The model under review builds one solid part; all positions refer to its coordinate system, in mm. A direction names the side the tool comes from. Round coordinates to 2 decimals unless told otherwise and drop trailing zeros. Order: outer loops, then holes, each group sorted by start corner. A loop starts at its lowest first (then second) coordinate and runs counter-clockwise, first axis right, second up. Notation, with made-up numbers: M 29.5,29.5 L 39.5,29.5 A17 ccw 39.5,45.5 Z; hole C 66,50.25 d1. An arc over 180 degrees is marked long. Use a Markdown table: item, result. Add a question column.
1. The part is to be moulded in two halves that separate along X. For faces 1 (the cylindrical face through (105.86, 32.29, 1.62)), 2 (the flat face through (72, 50, 3.2)), 3 (the cylindrical face through (2.795, 79.649, 1.623)), 4 (the flat face through (145.885, 49, 2)), say which applies: +X half, -X half, draft (parallel to the pull), parting line (faces both ways), or undercut.
2. Consider section B-B on x = 53. State the section outline as (y, z) points (3 decimals).
3. Insertion check: P1, Ø1.4, axis at x = 85.34, y = 46.7, coming from the +Z side (3 decimals). The pin has a flat end and moves straight along its axis. Give the tip position at first contact, or say it passes through.
4. To check wall thickness, follow probe 1 along X at (y, z) = (14, 1.6); probe 2 along X at (y, z) = (56.5, 0.85); probe 3 along Y at (x, z) = (26, 2.65) (3 decimals). State the ranges of each line that lie inside material, in increasing order.
5. For faces 5 (the flat face through (0, 49, 2)), 6 (the flat face through (111, 95.25, 2)), 7 (the flat face through (24, 3.175, 2)), list the 3-axis set-ups (+Z, -Z, +X, -X, +Y, -Y) from which the entire face can be reached by the end or side of a thin tool; tool diameter is ignored.
6. Consider section A-A on y = 8. State the section outline as (x, z) points, then the cut area to 3 significant figures.
7. Consider section C-C on z = 2.5. Count the separate pieces of the cut face and the enclosed holes in it, then the cut area to 3 significant figures.
from build123d import *

# Parameters (mm, degrees)
SKETCH1_W           = 145.885353282
SKETCH1_H           = 98.425
BOSS_EXTRUDE1_DEPTH = 3.2004
SKETCH4_W           = 57.100000132
SKETCH4_H           = 31.75
CUT_EXTRUDE1_DEPTH  = 3.2004
SKETCH5_R           = 2.159
CUT_EXTRUDE2_DEPTH  = 3.2004
SKETCH7_R           = 1.1303
CUT_EXTRUDE3_DEPTH  = 3.2004
SKETCH9_W           = 7.62
SKETCH9_H           = 3.175
CUT_EXTRUDE5_DEPTH  = 3.2004
SKETCH10_R          = 0.59563
CUT_EXTRUDE6_DEPTH  = 3.2004
FILLET1_R           = 0.762
SKETCH11_R          = 1.7272
CUT_EXTRUDE7_DEPTH  = 3.2004


with BuildPart() as part:
    # Sketch1 → Boss-Extrude1 (new body)
    with BuildSketch(Plane.XY):
        with Locations((72.942676641, 49.2125)):
            Rectangle(SKETCH1_W, SKETCH1_H)
    extrude(amount=BOSS_EXTRUDE1_DEPTH)

    # Sketch4 → Cut-Extrude1 (cut)
    with BuildSketch(Plane.XY.offset(3.2004)):
        with Locations((56.982760066, 15.875)):
            Rectangle(SKETCH4_W, SKETCH4_H)
    extrude(amount=-CUT_EXTRUDE1_DEPTH, mode=Mode.SUBTRACT)

    # Sketch5 → Cut-Extrude2 (cut)
    with BuildSketch(Plane.XY.offset(3.2004)):
        with Locations((141.376853282, 80.9625)):
            Circle(SKETCH5_R)
        with Locations((141.376853282, 17.4625)):
            Circle(SKETCH5_R)
        with Locations((4.5085, 17.4625)):
            Circle(SKETCH5_R)
        with Locations((4.5085, 80.9625)):
            Circle(SKETCH5_R)
    extrude(amount=-CUT_EXTRUDE2_DEPTH, mode=Mode.SUBTRACT)

    # Sketch7 → Cut-Extrude3 (cut)
    with BuildSketch(Plane(origin=(0, 0, 0), x_dir=(-1, 0, 0), z_dir=(0, 0, -1))):
        with Locations((-59.937161658, 67.017728802)):
            Circle(SKETCH7_R)
        with Locations((-59.937161658, 46.697728802)):
            Circle(SKETCH7_R)
        with Locations((-85.337161658, 46.697728802)):
            Circle(SKETCH7_R)
        with Locations((-85.337161658, 67.017728802)):
            Circle(SKETCH7_R)
    extrude(amount=-CUT_EXTRUDE3_DEPTH, mode=Mode.SUBTRACT)

    # Sketch9 → Cut-Extrude5 (cut)
    with BuildSketch(Plane.XY.offset(3.2004)):
        with Locations((110.993373282, 96.8375)):
            Rectangle(SKETCH9_W, SKETCH9_H)
        with Locations((110.993373282, 1.5875)):
            Rectangle(SKETCH9_W, SKETCH9_H)
        with Locations((24.62276, 1.5875)):
            Rectangle(SKETCH9_W, SKETCH9_H)
    extrude(amount=-CUT_EXTRUDE5_DEPTH, mode=Mode.SUBTRACT)

    # Sketch10 → Cut-Extrude6 (cut)
    with BuildSketch(Plane.XY.offset(3.2004)):
        with Locations((98.232760132, 24.47)):
            Circle(SKETCH10_R)
        with Locations((134.232760132, 24.47)):
            Circle(SKETCH10_R)
        with Locations((98.232760132, 3.47)):
            Circle(SKETCH10_R)
        with Locations((134.232760132, 3.47)):
            Circle(SKETCH10_R)
    extrude(amount=-CUT_EXTRUDE6_DEPTH, mode=Mode.SUBTRACT)

    # Fillet1
    fillet1_edges = [part.edges().sort_by_distance(p)[0] for p in [
        (85.532760132, 0, 1.6002),
        (0, 98.425, 1.6002),
        (145.885353282, 98.425, 1.6002),
        (145.885353282, 0, 1.6002),
        (0, 0, 1.6002),
        (114.803373282, 98.425, 1.6002),
        (107.183373282, 98.425, 1.6002),
        (114.803373282, 0, 1.6002),
        (107.183373282, 0, 1.6002),
        (28.43276, 3.175, 1.6002),
        (20.81276, 0, 1.6002),
    ]]
    fillet(fillet1_edges, radius=FILLET1_R)

    # Sketch11 → Cut-Extrude7 (cut)
    with BuildSketch(Plane.XY.offset(3.2004)):
        with Locations((13.252676641, 55.5625)):
            Circle(SKETCH11_R)
        with Locations((13.252676641, 80.9625)):
            Circle(SKETCH11_R)
        with Locations((132.632676641, 55.5625)):
            Circle(SKETCH11_R)
        with Locations((132.632676641, 80.9625)):
            Circle(SKETCH11_R)
        with Locations((107.232676641, 33.3375)):
            Circle(SKETCH11_R)
        with Locations((94.532676641, 33.3375)):
            Circle(SKETCH11_R)
    extrude(amount=-CUT_EXTRUDE7_DEPTH, mode=Mode.SUBTRACT)


solid = part.part
Answer block:
| question | item | result |
|---|---|---|
| 1 | face 1 | undercut |
| 1 | face 2 | draft |
| 1 | face 3 | undercut |
| 1 | face 4 | +X half |
| 2 | outline | M 31.75,0 L 98.425,0 L 98.425,3.2 L 31.75,3.2 Z |
| 3 | P1 | through |
| 4 | probe 1 | 0 to 28.43, 85.53 to 145.89 |
| 4 | probe 2 | 0 to 11.8, 14.7 to 131.18, 134.08 to 145.89 |
| 4 | probe 3 | 3.175 to 98.425 |
| 5 | face 5 | +Z, -Z, -X, +Y, -Y |
| 5 | face 6 | +Z, -Z, +Y |
| 5 | face 7 | +Z, -Z, -Y |
| 6 | outline | M 0,0 L 28.43,0 L 28.43,3.2 L 0,3.2 Z; M 85.53,0 L 145.89,0 L 145.89,3.2 L 85.53,3.2 Z |
| 6 | area | 284 mm^2 |
| 7 | separate pieces | 1 |
| 7 | enclosed holes | 18 |
| 7 | area | 12,300 mm^2 |
